Source: CAD feature listing. Evaluate the final solid. Frame: model axes, mm. A direction names the side the tool comes from. Round coordinates to 2 decimals unless told otherwise and drop trailing zeros. Loops run counter-clockwise (first coordinate to the right, second up) from the corner with the lowest first, then second, coordinate; pieces in that order, holes last.
Item 1: Section query D-D on z = 1. Return loops of the section in (x, y), then the cut area to 3 significant figures.
Item 2: Access query for faces 1 (the flat face through (8, -8, -3)), 2 (the flat face through (15, 0, -2)), 3 (the cylindrical face through (17.71, 10.18, -3.48)). Directions: +Z, -Z, +X, -X, +Y, -Y. A direction counts if a zero-diameter tool reaches every point of the face in a straight line with its end or side. Return the directions, or none.
Item 3: Ray query, L1, parallel to Y at x = 19, z = -3.85; L2, parallel to Y at x = 2.3, z = 1; L3, parallel to Z at x = 1.6, y = -8. Return the intervals inside material, ascending.
Item 4: Section query B-B on x = 23. Return loops of the section in (y, z).
Item 5: Pull-direction query (Y, two-part tool) for faces 4 (the flat face through (0, 0, 0)), 5 (the flat face through (8, 8, -3)); classes: released by +Y, released by -Y, zero draft, split by the parting line, or undercut.
Item 6: First-contact query: P1, Ø2, axis at y = 8, z = 1, coming from the -X side; P2, Ø2, axis at x = 23.5, y = -3, coming from the +Z side; P3, Ø1, axis at x = 10, y = -8.5, coming from the +Z side; P4, Ø6, axis at y = 10.5, z = -2, coming from the -X side. Flat tips, straight axial feed; report the tip coordinate or a pass-through.
Item 7: Section query A-A on z = -3.75. Return loops of the section in (x, y), then the cut area to 3 significant figures.
Item 8: Section query C-C on y = 0. Return loops of the section in (x, z), then the cut area to 3 significant figures.
Autodesk Inventor part; units mm, degrees
ref_plane "YZ Plane" through (0, 0, 0) normal (1, 0, 0) x (0, 1, 0)
ref_plane "XZ Plane" through (0, 0, 0) normal (0, 1, 0) x (-1, 0, 0)
ref_plane "XY Plane" through (0, 0, 0) normal (0, 0, 1) x (1, 0, 0)
sketch "Sketch1" plane through (0, 0, 0) normal (1, 0, 0) x (0, 1, 0)
  point P0 (0, 0)
sketch "Sketch2" plane through (0, 0, 0) normal (1, 0, 0) x (0, 1, 0)
  line L0 (15, 5) -> (-15, 5)
  line L1 (-15, 5) -> (-15, -5)
  line L2 (-15, -5) -> (15, -5)
  line L3 (15, -5) -> (15, 5)
  point P0 (0, 0)
  dimension "d0" = 10
  dimension "d1" = 30
  dimension "d2" = 15
  dimension "d3" = 5
extrude "Extrusion1" add sketch "Sketch2" along normal blind 3
sketch "Sketch3" plane through (3, 0, 0) normal (1, 0, 0) x (0, 0, -1)
  line L0 (5, -15) -> (5, 15)
  line L1 (-5, -15) -> (5, -15)
  line L2 (5, 15) -> (2, 15)
  line L3 (2, 15) -> (2, -15)
  line L4 (2, -15) -> (5, -15)
  line L5 (5, -15) -> (5, 15)
  dimension "d16" = 3
sketch "Sketch4" plane through (0, 0, 0) normal (-1, 0, 0) x (0, 0, 1)
  circle A0 centre (1, 8) radius 1.75
  line L0 (5, 15) -> (5, -15)
  line L1 (-5, 15) -> (5, 15)
  dimension "d19" = 4
  dimension "d23" = 3.5
  dimension "d27" = 7
extrude "Extrusion4" add sketch "Sketch3" along normal blind 25
extrude "Extrusion5" cut sketch "Sketch4" against normal blind 25
mirror "Mirror1" about plane through (0, 0, 0) normal (0, 1, 0) of "Extrusion5"
sketch "Sketch5" plane through (3, -15, -2) normal (0, 0, 1) x (1, 0, 0)
  line L0 (0, 30) -> (0, 0)
  line L1 (0, 24.75) -> (10, 24.75)
  line L2 (10, 24.75) -> (10, 21.25)
  line L3 (10, 21.25) -> (0, 21.25)
  line L4 (0, 21.25) -> (0, 24.75)
  line L5 (0, 30) -> (25, 30)
  point P0 (-3, 15)
  point P1 (0, 21.25)
  dimension "d24" = 5.25
  dimension "d25" = 3.5
  dimension "d26" = 10
extrude "Extrusion6" cut sketch "Sketch5" against normal blind 1
fillet "Fillet2" radius 1.5 2 edges at (13, 9.75, -2.5) (13, 6.25, -2.5)
mirror "Mirror2" about plane through (0, 0, 0) normal (0, 1, 0) of "Extrusion6", "Fillet2"
sketch "Sketch6" plane through (3, -15, -2) normal (0, 0, 1) x (1, 0, 0)
  circle A0 centre (16, 24) radius 1.75
  circle A1 centre (20, 15) radius 1.75
  circle A2 centre (16, 6) radius 1.75
  line L0 (0, 30) -> (25, 30)
  line L1 (0, 0) -> (25, 0)
  line L2 (0, 30) -> (0, 0)
  line L3 (25, 30) -> (25, 0)
  point P0 (-3, 15)
  dimension "d31" = 3.5
  dimension "d32" = 3.5
  dimension "d33" = 3.5
  dimension "d34" = 6
  dimension "d35" = 6
  dimension "d36" = 15
  dimension "d40" = 9
  dimension "d41" = 5
  dimension "d42" = 9
extrude "Extrusion7" cut sketch "Sketch6" against normal blind 9 contours A0 | A1 | A2
properties part number "POUPLY_P4_V3"
Data:
1. outline: (0, -15) - (3, -15) - (3, -9.75) - (0, -9.75) - close; (0, -6.25) - (3, -6.25) - (3, 6.25) - (0, 6.25) - close; (0, 9.75) - (3, 9.75) - (3, 15) - (0, 15) - close
1. area: 69.0 mm2
2. face 1: +Z
2. face 2: +Z, +X, +Y, -Y
2. face 3: +Z, -Z
3. L1: y = -15 to -10.75, -7.25 to 7.25, 10.75 to 15
3. L2: y = -15 to -9.75, -6.25 to 6.25, 9.75 to 15
3. L3: z = -5 to -0.75, 2.75 to 5
4. outline: (-15, -5) - (-1.75, -5) - (-1.75, -2) - (-15, -2) - close; (1.75, -5) - (15, -5) - (15, -2) - (1.75, -2) - close
5. face 4: zero draft
5. face 5: undercut
6. P1: passes through
6. P2: stops at z = -2
6. P3: stops at z = -3
6. P4: stops at x = 0
7. outline: (0, -15) - (28, -15) - (28, 15) - (0, 15) - close; hole circle Ø3.5 at (19, -9); hole circle Ø3.5 at (19, 9); hole circle Ø3.5 at (23, 0)
7. area: 811 mm2
8. outline: (0, -5) - (21.25, -5) - (21.25, -2) - (3, -2) - (3, 5) - (0, 5) - close; (24.75, -5) - (28, -5) - (28, -2) - (24.75, -2) - close
8. area: 94.5 mm2
